```python
from build123d import *

# Parameters (mm, degrees)
SKETCH1_R           = 7.5
BOSS_EXTRUDE1_DEPTH = 55
FILLET1_R           = 2.54
BOSS_EXTRUDE2_DEPTH = 25
SKETCH4_R           = 7
CUT_EXTRUDE1_DEPTH  = 73.629195232
FILLET2_R           = 12
SKETCH5_R           = 2.5
CUT_EXTRUDE2_DEPTH  = 87.734978206


with BuildPart() as part:
    # Sketch1 → Boss-Extrude1 (new body)
    with BuildSketch(Plane.XY):
        with BuildLine():
            Line((-13.667840434, -6.5), (13.667840434, -6.5))
            ThreePointArc((13.667840434, -6.5), (32.373863542, 11.618950039), (25.5, -13.5))
            Line((25.5, -13.5), (-25.5, -13.5))
            ThreePointArc((-25.5, -13.5), (-32.373863542, 11.618950039), (-13.667840434, -6.5))
        make_face()
        with Locations((-25.5, 0)):
            Circle(SKETCH1_R, mode=Mode.SUBTRACT)
        with Locations(Location((25.5, 0, 0), (0, 0, 180))):
            Circle(SKETCH1_R, mode=Mode.SUBTRACT)
    extrude(amount=BOSS_EXTRUDE1_DEPTH)

    # Fillet1
    fillet1_edges = [part.edges().sort_by_distance(p)[0] for p in [
        (-13.667840434, -6.5, 27.5),
        (13.667840434, -6.5, 27.5),
    ]]
    fillet(fillet1_edges, radius=FILLET1_R)

    # Sketch2 → Boss-Extrude2 (add)
    with BuildSketch(Plane.XZ.offset(13.5)):
        Polygon((11, 15.637254902), (16, 10.245098039), (16, 55), (11, 55), align=None)
        Polygon((16, 0), (16, 10.245098039), (11, 15.637254902), (11, 0), align=None)
    extrude(amount=BOSS_EXTRUDE2_DEPTH)

    # Sketch4 → Cut-Extrude1 (cut, through all)
    with BuildSketch(Plane.XZ.offset(13.5)):
        with Locations((0, 27.5)):
            Circle(SKETCH4_R)
    extrude(amount=-CUT_EXTRUDE1_DEPTH, mode=Mode.SUBTRACT)

    # Fillet2
    fillet2_edges = [part.edges().sort_by_distance(p)[0] for p in [
        (13.5, -38.5, 0),
        (13.5, -38.5, 55),
    ]]
    fillet(fillet2_edges, radius=FILLET2_R)

    # Sketch5 → Cut-Extrude2 (cut, through all)
    with BuildSketch(Plane(origin=(11, 11.194119758, 4.468317801), x_dir=(0, 0, 1), z_dir=(-1, 0, 0))):
        with Locations(Location((11.781682199, -37.194119758, 0), (0, 0, 270))):
            Circle(SKETCH5_R)
        with Locations(Location((34.281682199, -37.194119758, 0), (0, 0, 270))):
            Circle(SKETCH5_R)
    extrude(amount=-CUT_EXTRUDE2_DEPTH, mode=Mode.SUBTRACT)


solid = part.part
```
Source: CAD feature listing. Evaluate the final solid. Frame: model axes, mm. A direction names the side the tool comes from. Give positions to 0.01 mm unless a question says otherwise; leave off trailing zeros. Order: outer loops, then holes, each group sorted by start corner. A loop starts at its lowest first (then second) coordinate and runs counter-clockwise, first axis right, second up.
(1) Pull-direction query (X, two-part tool) for faces 5 (the face through (-1.517, -10.049, 20.666)), 6 (the face through (13.465, -23.502, 16.36)), 7 (the face through (16, -26, 27)); classes: +X half, -X half, draft (parallel to the pull), parting line (faces both ways), or undercut.
(2) Access query for faces 1 (the face through (21, -13.5, 27)), 2 (the face through (11.942, -5.544, 27.885)), 3 (the face through (11, -26, 28)), 4 (the face through (4.29, -6.5, 33.23)). Directions: +Z, -Z, +X, -X, +Y, -Y. A direction counts if a zero-diameter tool reaches every point of the face in a straight line with its end or side. Return the directions, or none.
(3) Section query B-B (z = 27.5). Return the cut outline in (x, y).
(4) Section query A-A (x = 0). Return the cut outline in (y, z).
(5) Contact query for flat-ended pins moving along their axis: P1, Ø7.5, axis at y = -30, z = 32, coming from the +X side; P2, Ø6.5, axis at y = -26, z = 16.25, coming from the -X side; P3, Ø2, axis at x = -6.5, z = 34, coming from the +Y side. Output: stop coordinate, or through.
(6) Section query C-C (y = 2). Return the cut outline in (x, z).
(7) Material intervals for line 1 along Z through (x, y) = (14, -26); line 2 along X through (y, z) = (-1, 12.5); line 3 along X through (y, z) = (-4.5, 23.5), sorted ascending.
(8) Section query D-D (z = 38.75). Return the cut outline in (x, y).
Outcome:
1. face 5: undercut
1. face 6: draft
1. face 7: +X half
2. face 1: +Z, -Z, +X, -Y
2. face 2: +Z, -Z
2. face 3: +Z, -Z, -X, -Y
2. face 4: +Z, -Z, +Y
3. outline: (-25.5, -13.5) - (-7, -13.5) - (-7, -6.5) - (-9.96, -6.5) arc R2.54 cw to (-12.42, -3.33) arc R13.5 ccw (long way) to start; (7, -13.5) - (11, -13.5) - (11, -38.5) - (16, -38.5) - (16, -13.5) - (25.5, -13.5) arc R13.5 ccw (long way) to (12.42, -3.33) arc R2.54 cw to (9.96, -6.5) - (7, -6.5) - close; hole circle Ø15 at (-25.5, 0); hole circle Ø15 at (25.5, 0)
4. outline: (-13.5, 0) - (-6.5, 0) - (-6.5, 20.5) - (-13.5, 20.5) - close; (-13.5, 34.5) - (-6.5, 34.5) - (-6.5, 55) - (-13.5, 55) - close
5. P1: stops at x = 16
5. P2: stops at x = 11
5. P3: stops at y = -6.5
6. outline: (-38.85, 0) - (-32.73, 0) - (-32.73, 55) - (-38.85, 55) - close; (-18.27, 0) - (-12.15, 0) - (-12.15, 55) - (-18.27, 55) - close; (12.15, 0) - (18.27, 0) - (18.27, 55) - (12.15, 55) - close; (32.73, 0) - (38.85, 0) - (38.85, 55) - (32.73, 55) - close
7. line 1: z = 0 to 13.75, 18.75 to 36.25, 41.25 to 55
7. line 2: x = -38.96 to -32.93, -18.07 to -12.04, 12.04 to 18.07, 32.93 to 38.96
7. line 3: x = -38.23 to -31.5, -19.5 to -12.44, 12.44 to 19.5, 31.5 to 38.23
8. outline: (-25.5, -13.5) - (11, -13.5) - (11, -23.5) - (16, -23.5) - (16, -13.5) - (25.5, -13.5) arc R13.5 ccw (long way) to (12.42, -3.33) arc R2.54 cw to (9.96, -6.5) - (-9.96, -6.5) arc R2.54 cw to (-12.42, -3.33) arc R13.5 ccw (long way) to start; (11, -38.5) - (16, -38.5) - (16, -28.5) - (11, -28.5) - close; hole circle Ø15 at (-25.5, 0); hole circle Ø15 at (25.5, 0)
